The listing builds one solid part. Answer for the finished solid, in the listing's coordinates (mm). A direction names the side the tool comes from. Coordinates: 2 decimals unless noted, no trailing zeros. Order: outer loops, then holes, each group sorted by start corner. A loop starts at its lowest first (then second) coordinate and runs counter-clockwise, first axis right, second up. Notation, with made-up numbers: (-34, -7) -> (-16, -7) arc R16 cw to (-16, 19) -> close; hole circle Ø11 at (-22.5, 30.5). An arc over 180 degrees is marked (long way). Write each question's results on one line, items separated by ' | '. Start each with the question number.
(1) The part is cut by section B-B, the plane y = 34.5. Give the vertices of the cut face in (x, z), then the cut area to 3 significant figures.
(2) The part is cut by section C-C, the plane x = 57. Give the vertices of the cut face in (y, z).
(3) The part is cut by section A-A, the plane x = 75.27. Give the vertices of the cut face in (y, z).
(4) The part is cut by section D-D, the plane y = 61. Give the vertices of the cut face in (x, z), then the cut area to 3 significant figures.
(5) Given pin 1 (5 mm diameter, centred on x = 7.27, y = 34.5, fed in from +Z); pin 2 (1.5 mm diameter, centred on x = 7.5, z = 4, fed in from +Y); pin 3 (21 mm diameter, centred on x = 21.5, y = 11, fed in from +Z), each flat-ended and moving along its own axis, determine where each tip first touches the part or whether it passes through.
(6) A tool of negligible diameter and unlimited length cuts with its end or side. For faces 4 (the face through (55, 2, 4)), 5 (the face through (110.54, 34, 3)), 6 (the face through (103, 20.394, 4)), 7 (the face through (6, 50.606, 3)), 8 (the face through (13.973, 23.141, 1.521)), from which of +Z, -Z, +X, -X, +Y, -Y can it reach the whole face along a straight path? Write none if from no direction.
(7) Determine the mould class of faces 1 (the face through (6, 18.394, 3)), 2 (the face through (73.79, 3.89, 1.48)), 3 (the face through (30.09, 68.72, 1.48)) for opening direction X: +X half, -X half, draft (parallel to the pull), parting line (faces both ways), or undercut.
(8) Straight lines are drawn through the part: L1, parallel to Y at x = 75.27, z = 1.4; L2, parallel to X at y = 20.5, z = 1.75; L3, parallel to X at y = 64.5, z = 0.9. For each, find the intervals that lie inside material, in ascending order.
```python
from build123d import *

# Parameters (mm, degrees)
SKETCH1_W                  = 110.54
SKETCH1_H                  = 69
BOSS_EXTRUDE1_DEPTH        = 3
F_3_2_3_2_DIAMETER_HOLE1_D = 3.2
SKETCH5_R                  = 2.25
BOSS_EXTRUDE2_DEPTH        = 10
CUT_EXTRUDE2_DEPTH         = 131.690824468
CUT_EXTRUDE1_DEPTH         = 131.690824468
FILLET1_R                  = 2.25
FILLET3_R                  = 4
BOSS_EXTRUDE3_DEPTH        = 3
M1_6_TAPPED_HOLE1_D        = 1.25
FILLET2_R                  = 2
SKETCH10_W                 = 13
SKETCH10_H                 = 69
CUT_EXTRUDE3_DEPTH         = 3
FILLET4_R                  = 1


# Some blends are built 0.0001 mm under size
with BuildPart() as part:
    # Sketch1 → Boss-Extrude1 (new body)
    with BuildSketch(Plane.XY):
        with Locations((55.27, 34.5)):
            Rectangle(SKETCH1_W, SKETCH1_H)
    extrude(amount=BOSS_EXTRUDE1_DEPTH)

    # Ø3.2 (3.2) Diameter Hole1 (through all)
    with Locations(Plane.XY.offset(3)):
        with Locations((35.27, 64.5), (75.27, 64.5), (103.27, 34.5), (75.27, 4.5), (35.27, 4.5), (7.27, 34.5)):
            Hole(F_3_2_3_2_DIAMETER_HOLE1_D / 2)

    # Sketch5 → Boss-Extrude2 (add)
    with BuildSketch(Plane.XY.offset(3)):
        with Locations(Location((2.2856, 48.3557, 0), (0, 0, 180))):
            Circle(SKETCH5_R)
        with Locations(Location((2.2856, 20.6443, 0), (0, 0, 180))):
            Circle(SKETCH5_R)
        with Locations(Location((107.8734, 48.3557, 0), (0, 0, 180))):
            Circle(SKETCH5_R)
        with Locations(Location((107.8734, 20.6443, 0), (0, 0, 180))):
            Circle(SKETCH5_R)
    extrude(amount=BOSS_EXTRUDE2_DEPTH)

    # Sketch6 → Cut-Extrude2 (cut, through all)
    with BuildSketch(Plane.XY.offset(3)):
        with BuildLine():
            Line((16.77, 47), (93.77, 47))
            ThreePointArc((93.77, 47), (96.598427125, 45.828427125), (97.77, 43))
            Line((97.77, 43), (97.77, 26))
            ThreePointArc((97.77, 26), (96.598427125, 23.171572875), (93.77, 22))
            Line((93.77, 22), (16.77, 22))
            ThreePointArc((16.77, 22), (13.941572875, 23.171572875), (12.77, 26))
            Line((12.77, 26), (12.77, 43))
            ThreePointArc((12.77, 43), (13.941572875, 45.828427125), (16.77, 47))
        make_face()
    extrude(amount=-CUT_EXTRUDE2_DEPTH, mode=Mode.SUBTRACT)

    # Sketch2 → Cut-Extrude1 (cut, through all)
    with BuildSketch(Plane.XY.offset(3)):
        Polygon((0, 69), (30, 69), (10, 50.6057), (0, 50.6057), align=None)
        Polygon((110.54, 69), (80.54, 69), (100.54, 50.6057), (110.54, 50.6057), align=None)
        Polygon((0, 0), (30, 0), (10, 18.3943), (0, 18.3943), align=None)
        Polygon((110.54, 0), (80.54, 0), (100.54, 18.3943), (110.54, 18.3943), align=None)
    extrude(amount=-CUT_EXTRUDE1_DEPTH, mode=Mode.SUBTRACT)

    # Fillet1
    fillet1_edges = [part.edges().sort_by_distance(p)[0] for p in [
        (110.54, 50.6057, 1.5),
        (100.54, 50.6057, 1.5),
        (0, 18.3943, 1.5),
        (10, 18.3943, 1.5),
        (110.54, 18.3943, 1.5),
        (100.54, 18.3943, 1.5),
        (0, 50.6057, 1.5),
        (10, 50.6057, 1.5),
    ]]
    fillet(fillet1_edges, radius=FILLET1_R)

    # Fillet3
    fillet3_edges = [part.edges().sort_by_distance(p)[0] for p in [
        (80.54, 69, 1.5),
        (30, 0, 1.5),
        (80.54, 0, 1.5),
        (30, 69, 1.5),
    ]]
    fillet(fillet3_edges, radius=FILLET3_R)

    # Sketch9 → Boss-Extrude3 (add)
    with BuildSketch(Plane.XY.offset(3)):
        with BuildLine():
            Line((10.64576534, 51.19962007), (28.851972729, 67.944142098))
            ThreePointArc((28.851972729, 67.944142098), (30.106569989, 68.726698834), (31.559744378, 69))
            Line((31.559744378, 69), (78.980255622, 69))
            ThreePointArc((78.980255622, 69), (80.433430011, 68.726698834), (81.688027271, 67.944142098))
            Line((81.688027271, 67.944142098), (99.89423466, 51.19962007))
            ThreePointArc((99.89423466, 51.19962007), (100.599945619, 50.759431906), (101.417356213, 50.6057))
            Line((101.417356213, 50.6057), (107.8734, 50.6057))
            Line((107.8734, 50.6057), (108.29, 50.6057))
            ThreePointArc((108.29, 50.6057), (109.880990258, 49.946690258), (110.54, 48.3557))
            Line((110.54, 48.3557), (110.54, 20.6443))
            ThreePointArc((110.54, 20.6443), (109.880990258, 19.053309742), (108.29, 18.3943))
            Line((108.29, 18.3943), (107.8734, 18.3943))
            Line((107.8734, 18.3943), (101.417356213, 18.3943))
            ThreePointArc((101.417356213, 18.3943), (100.599945619, 18.240568094), (99.89423466, 17.80037993))
            Line((99.89423466, 17.80037993), (81.688027271, 1.055857902))
            ThreePointArc((81.688027271, 1.055857902), (80.433430011, 0.273301166), (78.980255622, 0))
            Line((78.980255622, 0), (31.559744378, 0))
            ThreePointArc((31.559744378, 0), (30.106569989, 0.273301166), (28.851972729, 1.055857902))
            Line((28.851972729, 1.055857902), (10.64576534, 17.80037993))
            ThreePointArc((10.64576534, 17.80037993), (9.940054381, 18.240568094), (9.122643787, 18.3943))
            Line((9.122643787, 18.3943), (2.2856, 18.3943))
            Line((2.2856, 18.3943), (2.25, 18.3943))
            ThreePointArc((2.25, 18.3943), (0.659009742, 19.053309742), (0, 20.6443))
            Line((0, 20.6443), (0, 48.3557))
            ThreePointArc((0, 48.3557), (0.659009742, 49.946690258), (2.25, 50.6057))
            Line((2.25, 50.6057), (2.2856, 50.6057))
            Line((2.2856, 50.6057), (9.122643787, 50.6057))
            ThreePointArc((9.122643787, 50.6057), (9.940054381, 50.759431906), (10.64576534, 51.19962007))
        make_face()
        with BuildLine():
            Line((11.999651165, 49.727549021), (30.205858553, 66.472071049))
            ThreePointArc((30.205858553, 66.472071049), (30.833157184, 66.863349417), (31.559744378, 67))
            Line((31.559744378, 67), (78.980255622, 67))
            ThreePointArc((78.980255622, 67), (79.706842816, 66.863349417), (80.334141447, 66.472071049))
            Line((80.334141447, 66.472071049), (98.540348835, 49.727549021))
            ThreePointArc((98.540348835, 49.727549021), (99.873358425, 48.896082489), (101.417356213, 48.6057))
            Line((101.417356213, 48.6057), (107.8734, 48.6057))
            Line((107.8734, 48.6057), (108.29, 48.6057))
            ThreePointArc((108.29, 48.6057), (108.466776695, 48.532476695), (108.54, 48.3557))
            Line((108.54, 48.3557), (108.54, 20.6443))
            ThreePointArc((108.54, 20.6443), (108.466776695, 20.467523305), (108.29, 20.3943))
            Line((108.29, 20.3943), (107.8734, 20.3943))
            Line((107.8734, 20.3943), (101.417356213, 20.3943))
            ThreePointArc((101.417356213, 20.3943), (99.873358425, 20.103917511), (98.540348835, 19.272450979))
            Line((98.540348835, 19.272450979), (80.334141447, 2.527928951))
            ThreePointArc((80.334141447, 2.527928951), (79.706842816, 2.136650583), (78.980255622, 2))
            Line((78.980255622, 2), (31.559744378, 2))
            ThreePointArc((31.559744378, 2), (30.833157184, 2.136650583), (30.205858553, 2.527928951))
            Line((30.205858553, 2.527928951), (11.999651165, 19.272450979))
            ThreePointArc((11.999651165, 19.272450979), (10.666641575, 20.103917511), (9.122643787, 20.3943))
            Line((9.122643787, 20.3943), (2.2856, 20.3943))
            Line((2.2856, 20.3943), (2.25, 20.3943))
            ThreePointArc((2.25, 20.3943), (2.073223305, 20.467523305), (2, 20.6443))
            Line((2, 20.6443), (2, 48.3557))
            ThreePointArc((2, 48.3557), (2.073223305, 48.532476695), (2.25, 48.6057))
            Line((2.25, 48.6057), (2.2856, 48.6057))
            Line((2.2856, 48.6057), (9.122643787, 48.6057))
            ThreePointArc((9.122643787, 48.6057), (10.666641575, 48.896082489), (11.999651165, 49.727549021))
        make_face(mode=Mode.SUBTRACT)
    extrude(amount=BOSS_EXTRUDE3_DEPTH)

    # M1.6 Tapped Hole1 (through all)
    with Locations(Plane.XY.offset(13)):
        with Locations((2.2856, 48.3557), (2.2856, 20.6443), (107.8734, 48.3557), (107.8734, 20.6443)):
            Hole(M1_6_TAPPED_HOLE1_D / 2)

    # Fillet2
    # the kernel refuses this fillet: 2 mm, written as the material it adds along each edge
    with BuildSketch(Plane(origin=(4.521667977, 20.3943, 6), x_dir=(1, 0, 0), z_dir=(0, 0, -1))) as fillet2_piece_1:
        with BuildLine():
            CenterArc((1.636915369, -2), FILLET2_R, 90, 65.684260829)
            ThreePointArc((-0.18566503, -1.176470588), (-0.013574106, -0.600743482), (0, 0))
            Line((0, 0), (1.636915369, 0))
        make_face()
    extrude(amount=3)
    with BuildSketch(Plane(origin=(2, 22.876100314, 6), x_dir=(0.9896542066602442, -0.14347317254344985, 0), z_dir=(0, 0, -1))) as fillet2_piece_2:
        with BuildLine():
            CenterArc((1.741562948, -1.926875227), FILLET2_R, 105.541291059, 66.209834964)
            Line((-0.237745465, -1.639928882), (0, 0))
            ThreePointArc((0, 0), (0.602848713, -0.082265369), (1.205697426, 0))
        make_face()
    extrude(amount=3)
    with BuildSketch(Plane(origin=(105.637332023, 48.6057, 6), x_dir=(0.15588599188398633, -0.9877750541162424, 0), z_dir=(0, 0, -1))) as fillet2_piece_3:
        with BuildLine():
            CenterArc((1.720377932, 1.928676151), FILLET2_R, 188.968184481, 65.684260829)
            Line((-0.255172176, 1.616904167), (0, 0))
            ThreePointArc((0, 0), (0.595515438, 0.08023933), (1.191030876, 0))
        make_face()
    extrude(amount=3)
    with BuildSketch(Plane(origin=(108.54, 46.20671316, 6), x_dir=(-0.9999579138949993, 0.00917444487481441, 0), z_dir=(0, 0, -1))) as fillet2_piece_4:
        with BuildLine():
            CenterArc((1.98260893, -1.904693967), FILLET2_R, 107.759172143, 71.715163512)
            Line((-0.017306897, -1.886345077), (0, 0))
            ThreePointArc((0, 0), (0.686287707, -0.107219287), (1.372575413, 0))
        make_face()
    extrude(amount=3)
    with BuildSketch(Plane(origin=(105.637332023, 20.3943, 6), x_dir=(0.15588599188398633, 0.9877750541162424, 0), z_dir=(0, 0, -1)), Plane(origin=(4.521667977, 48.6057, 6), x_dir=(-0.1558859918839805, -0.9877750541162433, 0), z_dir=(0, 0, -1))) as fillet2_piece_5:
        with BuildLine():
            CenterArc((1.720377932, -1.928676151), FILLET2_R, 105.34755469, 65.684260829)
            Line((-0.255172176, -1.616904167), (0, 0))
            ThreePointArc((0, 0), (0.595515438, -0.08023933), (1.191030876, 0))
        make_face()
    extrude(amount=3)
    with BuildSketch(Plane(origin=(108.54, 22.79328684, 6), x_dir=(-0.9999579138949993, -0.00917444487481441, 0), z_dir=(0, 0, -1))) as fillet2_piece_6:
        with BuildLine():
            CenterArc((1.98260893, 1.904693967), FILLET2_R, 180.525664345, 71.715163512)
            Line((-0.017306897, 1.886345077), (0, 0))
            ThreePointArc((0, 0), (0.686287707, 0.107219287), (1.372575413, 0))
        make_face()
    extrude(amount=3)
    with BuildSketch(Plane(origin=(2, 46.123899686, 6), x_dir=(0, -1, 0), z_dir=(0, 0, -1))) as fillet2_piece_7:
        with BuildLine():
            CenterArc((1.657072613, -2), FILLET2_R, 90, 66.209834964)
            ThreePointArc((-0.172985235, -1.193223529), (-0.005078349, -0.608414638), (0, 0))
            Line((0, 0), (1.657072613, 0))
        make_face()
    extrude(amount=3)

    # Sketch10 → Cut-Extrude3 (cut)
    with BuildSketch(Plane.XY.offset(6)):
        with Locations((35.351972729, 34.5)):
            Rectangle(SKETCH10_W, SKETCH10_H)
        with Locations((75.188027271, 34.5)):
            Rectangle(SKETCH10_W, SKETCH10_H)
    extrude(amount=-CUT_EXTRUDE3_DEPTH, mode=Mode.SUBTRACT)

    # Fillet4
    fillet4_edges = [part.edges().sort_by_distance(p)[0] for p in [
        (81.688027271, 3.773118052, 4.5),
        (41.851972729, 0, 4.5),
        (41.851972729, 2, 4.5),
        (68.688027271, 0, 4.5),
        (68.688027271, 2, 4.5),
        (81.688027271, 1.055857902, 4.5),
        (28.851972729, 1.055857902, 4.5),
        (28.851972729, 3.773118052, 4.5),
        (28.851972729, 65.226881948, 4.5),
        (28.851972729, 67.944142098, 4.5),
        (81.688027271, 65.226881948, 4.5),
        (81.688027271, 67.944142098, 4.5),
        (68.688027271, 67, 4.5),
        (68.688027271, 69, 4.5),
        (41.851972729, 69, 4.5),
        (41.851972729, 67, 4.5),
    ]]
    fillet(fillet4_edges, radius=FILLET4_R - 0.0001)  # a hair under: the kernel refuses the full size


solid = part.part
```
Established:
1) outline: (0, 0) -> (5.67, 0) -> (5.67, 3) -> (2, 3) -> (2, 6) -> (0, 6) -> close; (8.87, 0) -> (12.77, 0) -> (12.77, 3) -> (8.87, 3) -> close; (97.77, 0) -> (101.67, 0) -> (101.67, 3) -> (97.77, 3) -> close; (104.87, 0) -> (110.54, 0) -> (110.54, 6) -> (108.54, 6) -> (108.54, 3) -> (104.87, 3) -> close | area: 69.4 mm^2
2) outline: (0, 0) -> (22, 0) -> (22, 3) -> (2, 3) -> (2, 6) -> (0, 6) -> close; (47, 0) -> (69, 0) -> (69, 6) -> (67, 6) -> (67, 3) -> (47, 3) -> close
3) outline: (0, 0) -> (2.9, 0) -> (2.9, 3) -> (0, 3) -> close; (6.1, 0) -> (22, 0) -> (22, 3) -> (6.1, 3) -> close; (47, 0) -> (62.9, 0) -> (62.9, 3) -> (47, 3) -> close; (66.1, 0) -> (69, 0) -> (69, 3) -> (66.1, 3) -> close
4) outline: (21.3, 0) -> (89.24, 0) -> (89.24, 6) -> (86.28, 6) -> (86.28, 3) -> (24.26, 3) -> (24.26, 6) -> (21.3, 6) -> close | area: 222 mm^2
5) pin 1: stops at z = 3 | pin 2: stops at y = 50.61 | pin 3: stops at z = 6
6) face 4: +Z, +X, -X | face 5: +Z, -Z, +X, +Y, -Y | face 6: +Z | face 7: +Z, -Z, -X, +Y | face 8: +Z, -Z
7) face 1: draft | face 2: undercut | face 3: -X half
8) L1: y = 0 to 2.9, 6.1 to 22, 47 to 62.9, 66.1 to 69 | L2: x = 0 to 1.68, 2.89 to 107.27, 108.48 to 110.54 | L3: x = 25.11 to 33.67, 36.87 to 73.67, 76.87 to 85.43
